Could you check a few things on this drawing? It's one solid part, dimensions in mm from its lowest x, y, z. Give positions to 0.01 mm unless a question says otherwise; leave off trailing zeros. Order: outer loops, then holes, each group sorted by start corner. A loop starts at its lowest first (then second) coordinate and runs counter-clockwise, first axis right, second up. Notation, with made-up numbers: M 5,-30 L 16,-30 A14 cw 16,-11 Z; hole C 66,-13.75 d8. An arc over 180 degrees is marked long. Use one line per item in the form item = value.
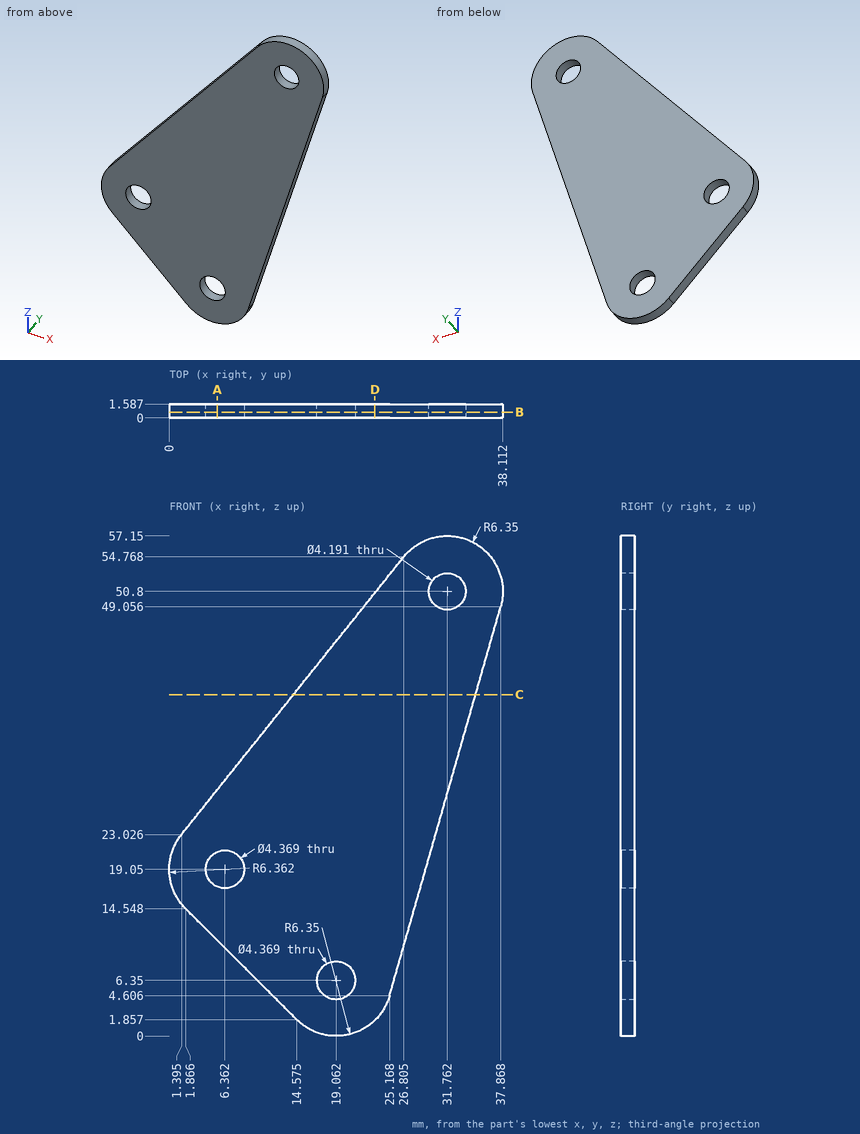
Q1. I'm going to push a flat-ended pin straight in: pin 1 Ø3.5 at (x, z) = (6.36, 19.05) entering from +Y. Where does the tip first touch, or does it pass through?
Found:
pin_1 = through
Q2. I need wall thicknesses on L1, parallel to X at y = 0.9, z = 52 (1 decimal); L2, parallel to Z at x = 6, y = 0.8 (1 decimal); L3, parallel to X at y = 0.2, z = 18.5 (1 decimal). Which ranges of each line are inside material? Lowest first, please.
Found:
L1 = 24.6 to 30, 33.5 to 38
L2 = 10.4 to 16.9, 21.2 to 28.8
L3 = 0 to 4.2, 8.5 to 29.1
Q3. I want a section at B-B on y = 0.65. State how many separate pieces and enclosed holes the cut face has, then the cut area to 3 significant figures.
Found:
separate_pieces = 1
enclosed_holes = 3
area = 1,110 mm²
Q4. I want a section at D-D on x = 23.5. Write out the boundary of the cut face in (y, z).
Found:
outline = M 0,1.81 L 1.59,1.81 L 1.59,50.64 L 0,50.64 Z
Q5. I want a section at C-C on z = 39. Write out the boundary of the cut face in (x, y) (1 decimal).
Found:
outline = M 14.2,0 L 35,0 L 35,1.6 L 14.2,1.6 Z
Q6. I want a section at A-A on x = 5.5. Write out the boundary of the cut face in (y, z).
Found:
outline = M 0,10.92 L 1.59,10.92 L 1.59,17.04 L 0,17.04 Z; M 0,21.06 L 1.59,21.06 L 1.59,28.15 L 0,28.15 Z
